For this review, take the finished solid that the model builds, in its own axes (mm). Face numbers are marked on the shaded views. A direction names the side the tool comes from. Coordinates: 2 decimals unless noted, no trailing zeros. Write each loop counter-clockwise with the first axis right and the second up, starting at its lowest first coordinate (ties: lowest second). Pieces come first, ordered by that corner, then holes.
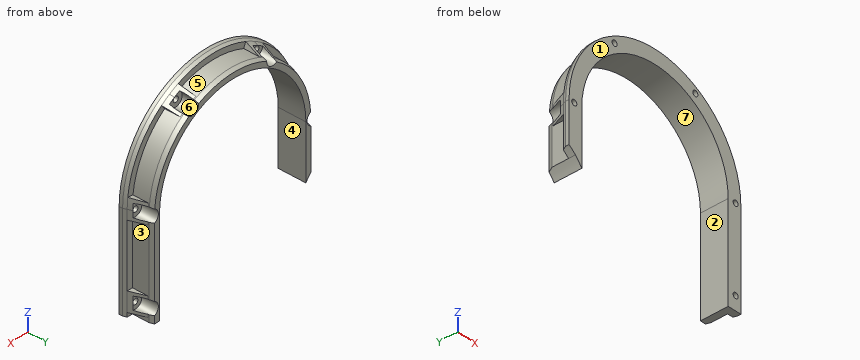
```python
from build123d import *
from OCP.BRepFilletAPI import BRepFilletAPI_MakeChamfer

# Parameters (mm, degrees)
BOSS_EXTRUDE1_DEPTH     = 25.4
BOSS_EXTRUDE2_DEPTH     = 6.35
CHAMFER1_SIZE           = 3.175
CHAMFER1_SIZE2          = 1.155605494
BOSS_EXTRUDE3_DEPTH     = 8.89
REVOLVE1_ANGLE          = 6.5
CHAMFER2_SIZE           = 3.81
CHAMFER2_SIZE2          = 1.386726593
CIRPATTERN1_COUNT       = 3
CIRPATTERN1_ANGLE       = 120
LPATTERN1_COUNT         = 2
LPATTERN1_PITCH         = 76.2
CUT_EXTRUDE1_DEPTH      = 258.62068172
CUT_EXTRUDE1_DEPTH_BACK = 258.62068172
SKETCH8_R               = 2.54
SKETCH8_3_R             = 6.35
CUT_EXTRUDE2_DEPTH      = 15.24


with BuildPart() as part:
    # Sketch2 → Boss-Extrude1 (new body)
    with BuildSketch(Plane(origin=(0, 0, 0), x_dir=(1, 0, 0), z_dir=(0, 1, 0))):
        with BuildLine():
            Line((186.055, 0), (186.055, -76.2))
            ThreePointArc((186.055, -76.2), (113.03, -149.225), (40.005, -76.2))
            Line((40.005, -76.2), (40.005, -25.840677236))
            ThreePointArc((40.005, -25.840677236), (37.038884837, -29.937629082), (33.655, -33.69690787))
            Line((33.655, -33.69690787), (33.655, -76.2))
            ThreePointArc((33.655, -76.2), (113.03, -155.575), (192.405, -76.2))
            Line((192.405, -76.2), (192.405, 12.7))
            Line((192.405, 12.7), (186.055, 12.7))
            Line((186.055, 12.7), (186.055, 0))
        make_face()
    extrude(amount=BOSS_EXTRUDE1_DEPTH)

    # Sketch2_3 → Boss-Extrude2 (add)
    with BuildSketch(Plane(origin=(0, 0, 0), x_dir=(1, 0, 0), z_dir=(0, 1, 0))):
        with BuildLine():
            Line((198.755, 12.7), (192.405, 12.7))
            Line((192.405, 12.7), (192.405, -76.2))
            ThreePointArc((192.405, -76.2), (113.03, -155.575), (33.655, -76.2))
            Line((33.655, -76.2), (33.655, -33.69690787))
            ThreePointArc((33.655, -33.69690787), (30.595993432, -36.496928788), (27.305, -39.020220399))
            Line((27.305, -39.020220399), (27.305, -76.2))
            ThreePointArc((27.305, -76.2), (113.03, -161.925), (198.755, -76.2))
            Line((198.755, -76.2), (198.755, 12.7))
        make_face()
    extrude(amount=BOSS_EXTRUDE2_DEPTH)

    # Chamfer1: one chamfer whose edges measure the first distance from different faces: ONE call of the kernel's chamfer builder (chamfer() names one face for all edges)
    chamfer1_edges_1 = [part.edges().sort_by_distance(p)[0] for p in [
        (198.755, 6.35, 31.75),
    ]]
    chamfer1_side_1 = [part.faces().sort_by_distance(p)[0] for p in [
        (198.755, 3.175, 31.75),
    ]]
    chamfer1_edges_2 = [part.edges().sort_by_distance(p)[0] for p in [
        (27.305, 6.35, 57.6101102),
    ]]
    chamfer1_side_2 = [part.faces().sort_by_distance(p)[0] for p in [
        (27.305, 3.175, 57.6101102),
    ]]
    chamfer1_edges_3 = [part.edges().sort_by_distance(p)[0] for p in [
        (113.03, 6.35, 161.925),
    ]]
    chamfer1_side_3 = [part.faces().sort_by_distance(p)[0] for p in [
        (113.03, 3.175, 161.925),
    ]]
    chamfer1 = BRepFilletAPI_MakeChamfer(part.part.solid().wrapped)
    for e in chamfer1_edges_1:
        chamfer1.Add(CHAMFER1_SIZE, CHAMFER1_SIZE2, e.wrapped, chamfer1_side_1[0].wrapped)  # the first distance lies on this face
    for e in chamfer1_edges_2:
        chamfer1.Add(CHAMFER1_SIZE, CHAMFER1_SIZE2, e.wrapped, chamfer1_side_2[0].wrapped)  # the first distance lies on this face
    for e in chamfer1_edges_3:
        chamfer1.Add(CHAMFER1_SIZE, CHAMFER1_SIZE2, e.wrapped, chamfer1_side_3[0].wrapped)  # the first distance lies on this face
    add(Compound.cast(chamfer1.Shape()), mode=Mode.REPLACE)

    # Chamfer2: one chamfer whose edges measure the first distance from different faces: ONE call of the kernel's chamfer builder (chamfer() names one face for all edges)
    chamfer2_edges_1 = [part.edges().sort_by_distance(p)[0] for p in [
        (113.03, 25.4, 155.575),
    ]]
    chamfer2_side_1 = [part.faces().sort_by_distance(p)[0] for p in [
        (113.03, 15.875, 155.575),
    ]]
    chamfer2_edges_2 = [part.edges().sort_by_distance(p)[0] for p in [
        (192.405, 25.4, 31.75),
    ]]
    chamfer2_side_2 = [part.faces().sort_by_distance(p)[0] for p in [
        (192.405, 15.875, 31.75),
    ]]
    chamfer2_edges_3 = [part.edges().sort_by_distance(p)[0] for p in [
        (33.655, 25.4, 54.948453935),
    ]]
    chamfer2_side_3 = [part.faces().sort_by_distance(p)[0] for p in [
        (33.655, 15.875, 54.948453935),
    ]]
    chamfer2 = BRepFilletAPI_MakeChamfer(part.part.solid().wrapped)
    for e in chamfer2_edges_1:
        chamfer2.Add(CHAMFER2_SIZE, CHAMFER2_SIZE2, e.wrapped, chamfer2_side_1[0].wrapped)  # the first distance lies on this face
    for e in chamfer2_edges_2:
        chamfer2.Add(CHAMFER2_SIZE, CHAMFER2_SIZE2, e.wrapped, chamfer2_side_2[0].wrapped)  # the first distance lies on this face
    for e in chamfer2_edges_3:
        chamfer2.Add(CHAMFER2_SIZE, CHAMFER2_SIZE2, e.wrapped, chamfer2_side_3[0].wrapped)  # the first distance lies on this face
    add(Compound.cast(chamfer2.Shape()), mode=Mode.REPLACE)


with BuildPart() as body_2:
    # Sketch4 → Boss-Extrude3 (new body)
    with BuildSketch(Plane.XY.offset(76.2)):
        Polygon((28.460605494, 6.35), (33.655, 20.621481614), (33.655, 6.35), align=None)
    extrude(amount=-BOSS_EXTRUDE3_DEPTH)


with BuildPart() as body_3:
    # Sketch4_4 → Revolve1 (revolve)
    with BuildSketch(Plane.XY.offset(76.2)):
        Polygon((28.460605494, 6.35), (33.655, 20.621481614), (33.655, 6.35), align=None)
    revolve(axis=Axis((113.03, 0, 76.2), (0, 1, 0)), revolution_arc=REVOLVE1_ANGLE)


with BuildPart() as body_4:
    # Mirror1: mirrored copy
    add(body_3.part.mirror(Plane.ZY.offset(-113.03)))


with BuildPart() as body_5:
    # Mirror1 2: mirrored copy
    add(body_2.part.mirror(Plane.ZY.offset(-113.03)))


with BuildPart() as cirpattern1_1:
    # CirPattern1: pattern copy
    add(body_3.part.rotate(Axis((113.03, 0, 76.2), (0, 1, 0)), 1 * CIRPATTERN1_ANGLE / (CIRPATTERN1_COUNT - 1)))


with BuildPart() as cirpattern1_2:
    # CirPattern1: pattern copy
    add(body_3.part.rotate(Axis((113.03, 0, 76.2), (0, 1, 0)), 2 * CIRPATTERN1_ANGLE / (CIRPATTERN1_COUNT - 1)))


with BuildPart() as body_8:
    # Mirror2: mirrored copy
    add(cirpattern1_1.part.mirror(Plane(origin=(56.515, 0, 174.08685139), x_dir=(-0.499999999999998, 0, 0.8660254037844398), z_dir=(0.8660254037844398, 0, 0.499999999999998))))


with BuildPart() as body_9:
    # Mirror3: mirrored copy
    add(cirpattern1_2.part.mirror(Plane(origin=(169.545, 0, 174.08685139), x_dir=(0.5000000000000039, 0, 0.8660254037844363), z_dir=(0.8660254037844363, 0, -0.500000000000004))))


with BuildPart() as lpattern1_1:
    # LPattern1: pattern copy
    add(body_5.part.moved(Location(Vector(0, 0, -1) * (1 * LPATTERN1_PITCH))))


with BuildPart() as body_11:
    # Mirror4: mirrored copy
    add(lpattern1_1.part.mirror(Plane(origin=(226.06, 0, 0), x_dir=(1, 0, 0), z_dir=(0, 0, -1))))


with BuildPart() as body_4_1:
    add(body_4.part)

    # Combine2: union body 8, body 11, body 5, CirPattern1_1, CirPattern1_2, part, body 9, body 2, LPattern1_1, body 3
    add(body_8.part)
    add(body_11.part)
    add(body_5.part)
    add(cirpattern1_1.part)
    add(cirpattern1_2.part)
    add(part.part)
    add(body_9.part)
    add(body_2.part)
    add(lpattern1_1.part)
    add(body_3.part)

    # Sketch8 → Cut-Extrude1 (cut, two sides: drawn at the far end of the back side and taken through both)
    with BuildSketch(Plane(origin=(0, 25.4, 0), x_dir=(1, 0, 0), z_dir=(0, 1, 0)).offset(-CUT_EXTRUDE1_DEPTH_BACK)):
        with Locations(Location((32.501726593, -76.2, 0), (0, 0, 270))):
            Circle(SKETCH8_R)
        with Locations(Location((72.765863296, -145.939530494, 0), (0, 0, 270))):
            Circle(SKETCH8_R)
        with Locations(Location((153.294136704, -145.939530494, 0), (0, 0, 270))):
            Circle(SKETCH8_R)
        with Locations(Location((193.558273407, -76.2, 0), (0, 0, 270))):
            Circle(SKETCH8_R)
        with Locations(Location((193.558273407, 0, 0), (0, 0, 270))):
            Circle(SKETCH8_R)
    extrude(amount=CUT_EXTRUDE1_DEPTH + CUT_EXTRUDE1_DEPTH_BACK, mode=Mode.SUBTRACT)

    # Sketch8_3 → Cut-Extrude2 (cut)
    with BuildSketch(Plane(origin=(0, 25.4, 0), x_dir=(1, 0, 0), z_dir=(0, 1, 0))):
        with Locations((32.501726593, -76.2)):
            Circle(SKETCH8_3_R)
        with Locations((72.765863296, -145.939530494)):
            Circle(SKETCH8_3_R)
        with Locations((153.294136704, -145.939530494)):
            Circle(SKETCH8_3_R)
        with Locations((193.558273407, -76.2)):
            Circle(SKETCH8_3_R)
        with Locations((193.558273407, 0)):
            Circle(SKETCH8_3_R)
    extrude(amount=-CUT_EXTRUDE2_DEPTH, mode=Mode.SUBTRACT)


solid = body_4_1.part
```
Q1. Add section A-A (z = 0). State the section outline as (x, y) points (3 decimals), then the cut area to 3 significant figures.
Ans:
outline: (186.055, 0) - (191.018, 0) - (191.018, 10.16) - (187.208, 10.16) - (187.208, 25.4) - (186.055, 25.4) - close; (196.098, 0) - (198.755, 0) - (198.755, 3.175) - (196.213, 10.16) - (196.098, 10.16) - close
area: 86.1 mm2
Q2. Tool access review of the marked faces 5, 6 and 7: name each direction out of +Z, -Z, +X, -X, +Y, -Y from which nothing blocks a thin tool from reaching the whole face with its end or side.
Ans:
face 5: +Z, +Y
face 6: +Y
face 7: -Z, +Y, -Y
Q3. Add section C-C (z = 54). State the section outline as (x, y) points (3 decimals), then the cut area to 3 significant figures.
Ans:
outline: (27.305, 0) - (40.005, 0) - (40.005, 25.4) - (35.042, 25.4) - (33.655, 21.59) - (33.655, 6.35) - (28.461, 6.35) - (27.305, 3.175) - close; (186.055, 0) - (198.755, 0) - (198.755, 3.175) - (197.599, 6.35) - (192.405, 6.35) - (192.405, 21.59) - (191.018, 25.4) - (186.055, 25.4) - close
area: 394 mm2
Q4. For probe 1 along X at (y, z) = (20.75, 28.5) (3 decimals); probe 2 along X at (y, z) = (14, 64) (3 decimals); probe 3 along X at (y, z) = (16.25, 22.5) (3 decimals), list the stretches that pass through material, from the lowest coordinate up.
Ans:
probe 1: x = 38.156 to 40.005, 186.055 to 192.405
probe 2: x = 33.655 to 40.005, 186.055 to 192.405
probe 3: x = 186.055 to 192.405
Q5. Add section B-B (x = 113.03). State the section outline as (y, z) points (3 decimals).
Ans:
outline: (0, 149.225) - (25.4, 149.225) - (25.4, 154.188) - (21.59, 155.575) - (6.35, 155.575) - (6.35, 160.769) - (3.175, 161.925) - (0, 161.925) - close
Q6. Draft analysis for pull direction X (two halves, no side actions). For the marked faces 1, 2, 3 and 4, state which applies: +X half, -X half, draft (parallel to the pull), parting line (faces both ways), or undercut.
Ans:
face 1: draft
face 2: undercut
face 3: +X half
face 4: undercut
Q7. Clearance check with flat-ended pins moving along their axes: pin 1 Ø1.5 at (y, z) = (5.5, 143.5) entering from -X; pin 2 Ø4 at (x, y) = (195.5, 12) entering from -Z; pin 3 Ø3 at (x, z) = (193.56, 76.2) entering from -Y; pin 4 Ø7.5 at (y, z) = (9, 37.5) entering from -X. State where each tip first meets the part, or that it passes through.
Ans:
pin 1: stops at x = 60.25
pin 2: stops at z = -8.89
pin 3: passes through
pin 4: stops at x = 28.1
